from build123d import *

# Parameters (mm, degrees)
SKETCH1_R           = 3.5
BOSS_EXTRUDE1_DEPTH = 16.5
SKETCH2_R           = 0.5
BOSS_EXTRUDE2_DEPTH = 4
SKETCH3_R           = 0.3
BOSS_EXTRUDE3_DEPTH = 3


with BuildPart() as part:
    # Sketch1 → Boss-Extrude1 (new body)
    with BuildSketch(Plane(origin=(0, 0, 0), x_dir=(1, 0, 0), z_dir=(0, 1, 0))):
        Circle(SKETCH1_R)
    extrude(amount=-BOSS_EXTRUDE1_DEPTH)

    # Sketch2 → Boss-Extrude2 (add)
    with BuildSketch(Plane(origin=(0, 0, 0), x_dir=(1, 0, 0), z_dir=(0, 1, 0))):
        Circle(SKETCH2_R)
    extrude(amount=BOSS_EXTRUDE2_DEPTH)

    # Sketch3 → Boss-Extrude3 (add)
    with BuildSketch(Plane.XZ.offset(16.5)):
        with Locations((2.5, 0)):
            Circle(SKETCH3_R)
        with Locations((-2.5, 0)):
            Circle(SKETCH3_R)
    extrude(amount=BOSS_EXTRUDE3_DEPTH)


solid = part.part
CAD build for the part. Positions are in the model's coordinates, mm. A direction names the side the tool comes from. Give positions to 0.01 mm unless a question says otherwise; leave off trailing zeros. Loops run counter-clockwise (first coordinate to the right, second up) from the corner with the lowest first, then second, coordinate; pieces in that order, holes last. Notation, with made-up numbers: M 5.5,35 L 45.5,35 A18 ccw 45.5,50 Z; hole C 85.25,39.25 d1. An arc over 180 degrees is marked long. Answer in a Markdown table with one row per item. Add a question column.
Item 1: Tool access for faces 1 (the face through (0, 4, 0)), 2 (the face through (-0.108, 1.972, 0.488)): list every direction of +Z, -Z, +X, -X, +Y, -Y with a clear straight run to the whole face (end or side of a thin tool).
Item 2: Drop flat-ended pins along their axis: P1, Ø4, axis at y = -3, z = -2, coming from the +X side; P2, Ø3.5, axis at x = 0, z = 1.5, coming from the -Y side; P3, Ø1.5, axis at y = -1, z = -1, coming from the -X side; P4, Ø1.5, axis at y = -9, z = -2, coming from the +X side. Give the stop position or say it passes through.
Item 3: Band-saw the part on D-D on x = -2.5. Give the cut face in (y, z), then the cut area to 3 significant figures.
Item 4: Probe probe 1 along Y at (x, z) = (-2.75, -1.25); probe 2 along X at (y, z) = (-2.5, 0.75); probe 3 along Z at (x, y) = (-3, -0.25). List the from-to ranges inside material, lowest first.
Item 5: Band-saw the part on A-A on x = 0. Give the cut face in (y, z), then the cut area to 4 significant figures.
Item 6: Band-saw the part on C-C on z = -3. Give the cut face in (x, y), then the cut area to 3 significant figures.
Item 7: Band-saw the part on B-B on y = 0.75. Give the cut face in (x, z), then the cut area to 3 significant figures.
Reply:
| question | item | result |
|---|---|---|
| 1 | face 1 | +Z, -Z, +X, -X, +Y |
| 1 | face 2 | +Y |
| 2 | P1 | stops at x = 3.5 |
| 2 | P2 | stops at y = -16.5 |
| 2 | P3 | stops at x = -3.49 |
| 2 | P4 | stops at x = 3.27 |
| 3 | outline | M -19.5,-0.3 L -16.5,-0.3 L -16.5,-2.45 L 0,-2.45 L 0,2.45 L -16.5,2.45 L -16.5,0.3 L -19.5,0.3 Z |
| 3 | area | 82.6 mm^2 |
| 4 | probe 1 | y = -16.5 to 0 |
| 4 | probe 2 | x = -3.42 to 3.42 |
| 4 | probe 3 | z = -1.8 to 1.8 |
| 5 | outline | M -16.5,-3.5 L 0,-3.5 L 0,-0.5 L 4,-0.5 L 4,0.5 L 0,0.5 L 0,3.5 L -16.5,3.5 Z |
| 5 | area | 119.5 mm^2 |
| 6 | outline | M -1.8,-16.5 L 1.8,-16.5 L 1.8,0 L -1.8,0 Z |
| 6 | area | 59.5 mm^2 |
| 7 | outline | C 0,0 d1 |
| 7 | area | 0.785 mm^2 |
